Can you work these out from the model? Positions are in its coordinate system, mm. Round coordinates to 2 decimals unless told otherwise and drop trailing zeros. Write each loop counter-clockwise with the first axis right and the second up, starting at its lowest first coordinate (ties: lowest second). Pieces come first, ordered by that corner, then holes. Notation, with made-up numbers: M -17.75,37.5 L 8.25,37.5 A18 cw 8.25,64.5 Z; hole C -15,16 d10. An arc over 180 degrees is marked long. Answer in a Markdown table with one row per item. Add a question column.
(1) Suppose I cut it at A-A, the plane z = 0.95. Write out the boundary of the cut face in (x, y).
(2) If I drill on probe 1 along X at (y, z) = (-58.5, 0.55); probe 2 along X at (y, z) = (118, 0.75); probe 3 along X at (y, z) = (-59.5, 0.7), over which ranges is the centre line in solid material (lowest first)?
(3) I'm going to push flat-ended pins straight in: pin 1 (1.9 mm diameter, centred on x = -10, y = -48.11, fed in from +Z); pin 2 (1.5 mm diameter, centred on x = -5, z = 0.5, fed in from +Y). Where does each tip first touch, or does it pass through?
from build123d import *

# Parameters (mm, degrees)
SKETCH_2_W               = 18
SKETCH_2_H               = 90
SKETCH_2_R               = 1.6
EXTRUDE_1_DEPTH          = 3
SKETCH_3_R               = 1.5
SKETCH_3_W               = 18
SKETCH_3_H               = 45
EXTRUDE_2_DEPTH          = 3
SKETCH_4_R               = 1.6
CUT_EXTRUDE_1_DEPTH      = 3
CUT_EXTRUDE_2_DEPTH      = 139.102072216
CUT_EXTRUDE_2_DEPTH_BACK = 3


with BuildPart() as part:
    # 草图2 → 凸台-拉伸1 (new body)
    with BuildSketch(Plane.XY):
        with Locations((-9, -88.108866795)):
            Rectangle(SKETCH_2_W, SKETCH_2_H)
        with Locations((-10, -125.108866795)):
            Circle(SKETCH_2_R, mode=Mode.SUBTRACT)
    extrude(amount=EXTRUDE_1_DEPTH)

    # 草图3 → 凸台-拉伸2 (add)
    # profile 1 of 2: a face of its own
    with BuildSketch(Plane.XY.offset(3)):
        Polygon((-18, 1.891133205), (0, 1.891133205), (0, 46.891133205), (0, 136.891133205), (-18, 136.891133205), (-18, 46.891133205), align=None)
        with Locations((-10, 128.891133205)):
            Circle(SKETCH_3_R, mode=Mode.SUBTRACT)
    # profile 2 of 2: a face of its own
    with BuildSketch(Plane.XY.offset(3)):
        with Locations((-9, -20.608866795)):
            Rectangle(SKETCH_3_W, SKETCH_3_H)
    extrude(amount=-EXTRUDE_2_DEPTH)

    # 草图4 → 切除-拉伸1 (cut)
    with BuildSketch(Plane.XY.offset(3)):
        with Locations((-10, -58.108866795)):
            Circle(SKETCH_4_R)
        with Locations((-10, -48.108866795)):
            Circle(SKETCH_4_R)
        with Locations((-10, 51.891133205)):
            Circle(SKETCH_4_R)
        with Locations((-10, 61.891133205)):
            Circle(SKETCH_4_R)
    extrude(amount=-CUT_EXTRUDE_1_DEPTH, mode=Mode.SUBTRACT)

    # 草图5 → 切除-拉伸2 (cut, two sides: drawn at the far end of the back side and taken through both)
    with BuildSketch(Plane.XY.offset(3).offset(-CUT_EXTRUDE_2_DEPTH_BACK)):
        with BuildLine():
            Line((-4, -110.108866795), (-4, -125.108866795))
            ThreePointArc((-4, -125.108866795), (-10, -131.108866795), (-16, -125.108866795))
            Line((-16, -125.108866795), (-16, 128.891133205))
            ThreePointArc((-16, 128.891133205), (-10, 134.891133205), (-4, 128.891133205))
            Line((-4, 128.891133205), (-4, 113.891133205))
            ThreePointArc((-4, 113.891133205), (-3.472135955, 111.655065228), (-2, 109.891133205))
            ThreePointArc((-2, 109.891133205), (-0.527864045, 108.127201183), (0, 105.891133205))
            Line((0, 105.891133205), (0, 136.891133205))
            Line((0, 136.891133205), (-18, 136.891133205))
            Line((-18, 136.891133205), (-18, -133.108866795))
            Line((-18, -133.108866795), (0, -133.108866795))
            Line((0, -133.108866795), (0, -102.108866795))
            ThreePointArc((0, -102.108866795), (-0.527864045, -104.344934772), (-2, -106.108866795))
            ThreePointArc((-2, -106.108866795), (-3.472135955, -107.872798817), (-4, -110.108866795))
        make_face()
    extrude(amount=CUT_EXTRUDE_2_DEPTH + CUT_EXTRUDE_2_DEPTH_BACK, mode=Mode.SUBTRACT)


solid = part.part
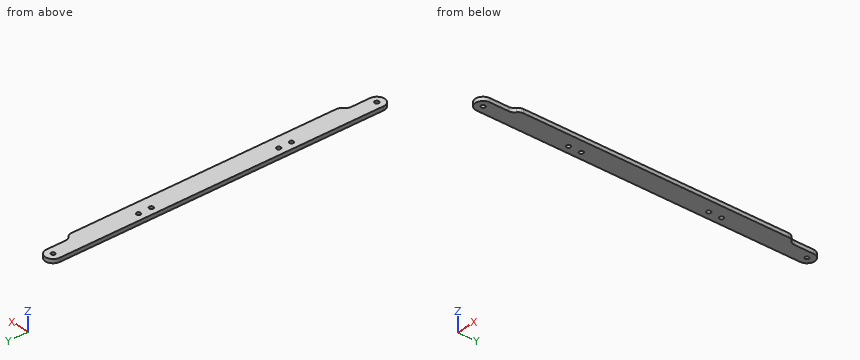
Calculated:
| question | item | result |
|---|---|---|
| 1 | outline | M -16,-125.11 A6 ccw -4,-125.11 L -4,-110.11 A5 cw -2,-106.11 A5 ccw 0,-102.11 L 0,105.89 A5 ccw -2,109.89 A5 cw -4,113.89 L -4,128.89 A6 ccw -16,128.89 Z; hole C -10,-125.11 d3.2; hole C -10,-58.11 d3.2; hole C -10,-48.11 d3.2; hole C -10,51.89 d3.2; hole C -10,61.89 d3.2; hole C -10,128.89 d3 |
| 2 | probe 1 | -16 to -11.55, -8.45 to 0 |
| 2 | probe 2 | -16 to -4 |
| 2 | probe 3 | -16 to -10.79, -9.21 to 0 |
| 3 | pin 1 | through |
| 3 | pin 2 | y = 133.13 |
